Read the model definition and answer for the solid it produces. Units are mm, in the model's axes. Give positions to 0.01 mm unless a question says otherwise; leave off trailing zeros. Write each loop counter-clockwise with the first axis right and the second up, starting at its lowest first coordinate (ties: lowest second). Pieces come first, ordered by that corner, then holes. Notation, with made-up numbers: (37.5, -21) -> (70.5, -21) arc R19 ccw to (70.5, 3) -> close; hole circle Ø5 at (7, 77.25). An arc over 180 degrees is marked (long way). Use a Markdown table: item, result.
from build123d import *

# Parameters (mm, degrees)
F0_R     = 3.175
F1_DEPTH = 228.6
F2_R     = 3.175
F3_DEPTH = 50.8
F4_R     = 6.35
F5_DEPTH = 6.35
F8_R     = 2.286
F9_DEPTH = 63.5


with BuildPart() as f1:
    # F0 (on Front) → F1 (new body)
    with BuildSketch(Plane.XZ):
        Circle(F0_R)
    extrude(amount=F1_DEPTH)

    # F2 (on Top) → F3 (join)
    with BuildSketch(Plane.XY):
        Circle(F2_R)
    extrude(amount=-F3_DEPTH)

    # F4 (on Right) → F5 (join, symmetric)
    with BuildSketch(Plane.YZ):
        Circle(F4_R)
    extrude(amount=F5_DEPTH, both=True)

    # F6 (on Right) → F7 (revolve)
    with BuildSketch(Plane.YZ):
        with BuildLine():
            Line((-228.6, 9.525), (-228.6, -9.525))
            ThreePointArc((-228.6, -9.525), (-219.075, 0), (-228.6, 9.525))
        make_face()
    revolve(axis=Axis((0, -228.6, 0), (0, 0, -1)))

    # F8 (on face) → F9 (cut, symmetric)
    with BuildSketch(Plane.YZ.offset(6.35)):
        Circle(F8_R)
    extrude(amount=F9_DEPTH, both=True, mode=Mode.SUBTRACT)


solid = f1.part
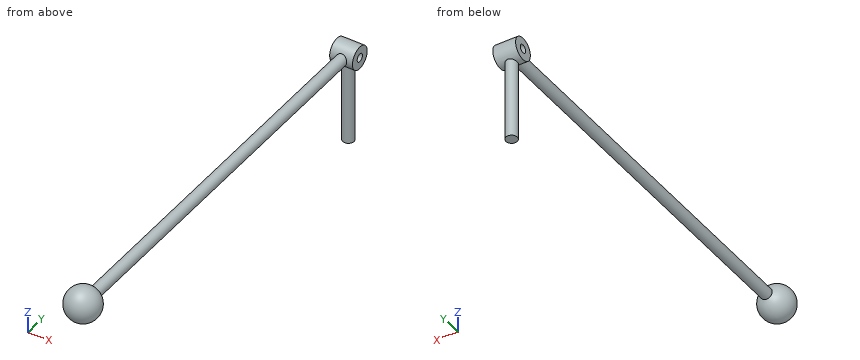
Item 1: Each of these flat-tipped pins is pushed along its axis until it touches: P1, Ø5.5, axis at y = 0, z = 0, coming from the -X side; P2, Ø14, axis at y = 0, z = 2.5, coming from the +X side; P3, Ø4, axis at y = 0, z = -1, coming from the -X side. Where does it stop, or does it pass through?
Return value:
| item | result |
|---|---|
| P1 | x = -6.35 |
| P2 | x = 6.35 |
| P3 | x = -6.35 |
Item 2: A cutting plane is placed at B-B (y = 0). Give the vertices of the cut face in (x, z) (3 decimals), then the cut area to 3 significant figures.
Return value:
| item | result |
|---|---|
| outline | (-6.35, -6.35) -> (-3.175, -6.35) -> (-3.175, -50.8) -> (3.175, -50.8) -> (3.175, -6.35) -> (6.35, -6.35) -> (6.35, -2.286) -> (-6.35, -2.286) -> close; (-6.35, 2.286) -> (6.35, 2.286) -> (6.35, 6.35) -> (-6.35, 6.35) -> close |
| area | 385 mm^2 |
Item 3: Straight lines are drawn through the part: line 1 along Z through (x, y) = (-3, 0); line 2 along Z through (x, y) = (-3.5, 0); line 3 along Y through (x, z) = (-0.5, -32). For each, find the intervals that lie inside material, in ascending order. Write a range as [from, to].
Return value:
| item | result |
|---|---|
| line 1 | [-50.8, -2.29], [2.29, 6.35] |
| line 2 | [-6.35, -2.29], [2.29, 6.35] |
| line 3 | [-3.14, 3.14] |
Item 4: A cutting plane is placed at A-A (z = 0). Give the vertices of the cut face in (x, y) (3 decimals).
Return value:
| item | result |
|---|---|
| outline | (-6.35, -6.35) -> (-3.175, -6.35) -> (-3.175, -219.62) arc R9.525 ccw (long way) to (3.175, -219.62) -> (3.175, -6.35) -> (6.35, -6.35) -> (6.35, -2.286) -> (-6.35, -2.286) -> close; (-6.35, 2.286) -> (6.35, 2.286) -> (6.35, 6.35) -> (-6.35, 6.35) -> close |
Item 5: A cutting plane is placed at D-D (z = -30). Give the vertices of the cut face in (x, y) (3 decimals), then the cut area to 3 significant figures.
Return value:
| item | result |
|---|---|
| outline | circle Ø6.35 at (0, 0) |
| area | 31.7 mm^2 |
Item 6: A cutting plane is placed at C-C (x = 0). Give the vertices of the cut face in (y, z) (3 decimals), then the cut area to 3 significant figures.
Return value:
| item | result |
|---|---|
| outline | (-219.62, -3.175) -> (-5.499, -3.175) arc R6.35 ccw to (-3.175, -5.499) -> (-3.175, -50.8) -> (3.175, -50.8) -> (3.175, -5.499) arc R6.35 ccw (long way) to (-5.499, 3.175) -> (-219.62, 3.175) arc R9.525 ccw (long way) to start; hole circle Ø4.572 at (0, 0) |
| area | 2,030 mm^2 |
